```python
from build123d import *
from OCP.BRepFilletAPI import BRepFilletAPI_MakeChamfer

# Parameters (mm, degrees)
SKETCH1_W               = 21
SKETCH1_H               = 36
SKETCH1_R               = 8.9
BOSS_EXTRUDE1_DEPTH     = 24
SKETCH1_2_R             = 8.9
BOSS_EXTRUDE2_DEPTH     = 27
SKETCH2_R               = 2
SKETCH2_R_2             = 1.3
CUT_EXTRUDE1_DEPTH      = 3
CHAMFER1_SIZE           = 4
CHAMFER1_SIZE2          = 2
CHAMFER2_SIZE           = 2
CHAMFER2_SIZE2          = 4
CUT_EXTRUDE2_DEPTH      = 32.784430151
CUT_EXTRUDE2_DEPTH_BACK = 32.784430151
SKETCH4_R               = 2
CUT_EXTRUDE3_DEPTH      = 39.65229618
CUT_EXTRUDE3_DEPTH_BACK = 39.65229618
SKETCH5_W               = 17
SKETCH5_H               = 12.551801511
SKETCH7_W               = 6
SKETCH7_H               = 6
BOSS_EXTRUDE3_DEPTH     = 1.5
BOSS_EXTRUDE4_START     = -21
SKETCH7_2_W             = 6
SKETCH7_2_H             = 6
BOSS_EXTRUDE4_DEPTH     = 1.5
CUT_EXTRUDE6_START      = 1.5
SKETCH6_R               = 2
CUT_EXTRUDE6_DEPTH      = 3
CUT_EXTRUDE7_START      = -19.5
SKETCH6_3_R             = 2
CUT_EXTRUDE7_DEPTH      = 3
SKETCH8_W               = 18
SKETCH8_H               = 10
CUT_EXTRUDE8_DEPTH      = 3
CUT_EXTRUDE9_START      = -21
SKETCH8_2_W             = 18
SKETCH8_2_H             = 10
CUT_EXTRUDE9_DEPTH      = 3


with BuildPart() as part:
    # Sketch1 → Boss-Extrude1 (new body)
    with BuildSketch(Plane.XY):
        Rectangle(SKETCH1_W, SKETCH1_H)
        with Locations((0, 9)):
            Circle(SKETCH1_R, mode=Mode.SUBTRACT)
    extrude(amount=BOSS_EXTRUDE1_DEPTH)

    # Sketch1<2> → Boss-Extrude2 (add)
    with BuildSketch(Plane.XY):
        with Locations((0, 9)):
            Circle(SKETCH1_2_R)
    extrude(amount=BOSS_EXTRUDE2_DEPTH)

    # Sketch2 → Cut-Extrude1 (cut)
    with BuildSketch(Plane.XY.offset(27)):
        with Locations((0, 15)):
            Circle(SKETCH2_R)
        with Locations((6, 9)):
            Circle(SKETCH2_R)
        with Locations((0, 3)):
            Circle(SKETCH2_R)
        with Locations((-6, 9)):
            Circle(SKETCH2_R)
        with Locations((0, 9)):
            Circle(SKETCH2_R_2)
    extrude(amount=-CUT_EXTRUDE1_DEPTH, mode=Mode.SUBTRACT)

    # Chamfer1: one chamfer whose edges measure the first distance from different faces: ONE call of the kernel's chamfer builder (chamfer() names one face for all edges)
    chamfer1_edges_1 = [part.edges().sort_by_distance(p)[0] for p in [
        (-10.5, -18, 12),
    ]]
    chamfer1_side_1 = [part.faces().sort_by_distance(p)[0] for p in [
        (-10.5, 0, 12),
    ]]
    chamfer1_edges_2 = [part.edges().sort_by_distance(p)[0] for p in [
        (10.5, 18, 12),
    ]]
    chamfer1_side_2 = [part.faces().sort_by_distance(p)[0] for p in [
        (10.5, 0, 12),
    ]]
    chamfer1 = BRepFilletAPI_MakeChamfer(part.part.solid().wrapped)
    for e in chamfer1_edges_1:
        chamfer1.Add(CHAMFER1_SIZE, CHAMFER1_SIZE2, e.wrapped, chamfer1_side_1[0].wrapped)  # the first distance lies on this face
    for e in chamfer1_edges_2:
        chamfer1.Add(CHAMFER1_SIZE, CHAMFER1_SIZE2, e.wrapped, chamfer1_side_2[0].wrapped)  # the first distance lies on this face
    add(Compound.cast(chamfer1.Shape()), mode=Mode.REPLACE)

    # Chamfer2: one chamfer whose edges measure the first distance from different faces: ONE call of the kernel's chamfer builder (chamfer() names one face for all edges)
    chamfer2_edges_1 = [part.edges().sort_by_distance(p)[0] for p in [
        (10.5, -18, 12),
    ]]
    chamfer2_side_1 = [part.faces().sort_by_distance(p)[0] for p in [
        (1, -18, 12),
    ]]
    chamfer2_edges_2 = [part.edges().sort_by_distance(p)[0] for p in [
        (-10.5, 18, 12),
    ]]
    chamfer2_side_2 = [part.faces().sort_by_distance(p)[0] for p in [
        (-1, 18, 12),
    ]]
    chamfer2 = BRepFilletAPI_MakeChamfer(part.part.solid().wrapped)
    for e in chamfer2_edges_1:
        chamfer2.Add(CHAMFER2_SIZE, CHAMFER2_SIZE2, e.wrapped, chamfer2_side_1[0].wrapped)  # the first distance lies on this face
    for e in chamfer2_edges_2:
        chamfer2.Add(CHAMFER2_SIZE, CHAMFER2_SIZE2, e.wrapped, chamfer2_side_2[0].wrapped)  # the first distance lies on this face
    add(Compound.cast(chamfer2.Shape()), mode=Mode.REPLACE)

    # Sketch4 → Cut-Extrude2 (cut, two sides: drawn at the far end of the back side and taken through both)
    with BuildSketch(Plane.XY.offset(24).offset(-CUT_EXTRUDE2_DEPTH_BACK)):
        with Locations((0, -15)):
            Circle(SKETCH4_R)
        with Locations((-6, -15)):
            Circle(SKETCH4_R)
        with Locations((6, -15)):
            Circle(SKETCH4_R)
    extrude(amount=CUT_EXTRUDE2_DEPTH + CUT_EXTRUDE2_DEPTH_BACK, mode=Mode.SUBTRACT)

    # Sketch5 → Cut-Extrude3 (cut, two sides: drawn at the far end of the back side and taken through both)
    with BuildSketch(Plane.ZY.offset(10.5).offset(-CUT_EXTRUDE3_DEPTH_BACK)):
        with Locations((12, -19.275900756)):
            Rectangle(SKETCH5_W, SKETCH5_H)
    extrude(amount=CUT_EXTRUDE3_DEPTH + CUT_EXTRUDE3_DEPTH_BACK, mode=Mode.SUBTRACT)

    # Sketch7 → Boss-Extrude3 (add)
    with BuildSketch(Plane(origin=(10.5, 0, 0), x_dir=(0, 0, -1), z_dir=(1, 0, 0))):
        with Locations((-18, 9)):
            Rectangle(SKETCH7_W, SKETCH7_H)
        with Locations((-6, 9)):
            Rectangle(SKETCH7_W, SKETCH7_H)
        with Locations((-6, -9)):
            Rectangle(SKETCH7_W, SKETCH7_H)
        with Locations((-18, -9)):
            Rectangle(SKETCH7_W, SKETCH7_H)
    extrude(amount=BOSS_EXTRUDE3_DEPTH)

    # Sketch7<2> → Boss-Extrude4 (add)
    with BuildSketch(Plane(origin=(10.5, 0, 0), x_dir=(0, 0, -1), z_dir=(1, 0, 0)).offset(BOSS_EXTRUDE4_START)):
        with Locations((-18, 9)):
            Rectangle(SKETCH7_2_W, SKETCH7_2_H)
        with Locations((-6, 9)):
            Rectangle(SKETCH7_2_W, SKETCH7_2_H)
        with Locations((-6, -9)):
            Rectangle(SKETCH7_2_W, SKETCH7_2_H)
        with Locations((-18, -9)):
            Rectangle(SKETCH7_2_W, SKETCH7_2_H)
    extrude(amount=-BOSS_EXTRUDE4_DEPTH)

    # Sketch6 → Cut-Extrude6 (cut)
    with BuildSketch(Plane(origin=(10.5, 0, 0), x_dir=(0, 0, -1), z_dir=(1, 0, 0)).offset(CUT_EXTRUDE6_START)):
        with Locations((-12, 9)):
            Circle(SKETCH6_R)
        with Locations((-6, 9)):
            Circle(SKETCH6_R)
        with Locations((-18, 9)):
            Circle(SKETCH6_R)
        with Locations((-12, -9)):
            Circle(SKETCH6_R)
        with Locations((-6, -9)):
            Circle(SKETCH6_R)
        with Locations((-18, -9)):
            Circle(SKETCH6_R)
    extrude(amount=-CUT_EXTRUDE6_DEPTH, mode=Mode.SUBTRACT)

    # Sketch6<3> → Cut-Extrude7 (cut)
    with BuildSketch(Plane(origin=(10.5, 0, 0), x_dir=(0, 0, -1), z_dir=(1, 0, 0)).offset(CUT_EXTRUDE7_START)):
        with Locations((-12, 9)):
            Circle(SKETCH6_3_R)
        with Locations((-6, 9)):
            Circle(SKETCH6_3_R)
        with Locations((-18, 9)):
            Circle(SKETCH6_3_R)
        with Locations((-12, -9)):
            Circle(SKETCH6_3_R)
        with Locations((-6, -9)):
            Circle(SKETCH6_3_R)
        with Locations((-18, -9)):
            Circle(SKETCH6_3_R)
    extrude(amount=-CUT_EXTRUDE7_DEPTH, mode=Mode.SUBTRACT)

    # Sketch8 → Cut-Extrude8 (cut)
    with BuildSketch(Plane(origin=(10.5, 0, 0), x_dir=(0, 0, -1), z_dir=(1, 0, 0))):
        with Locations((-12, 0)):
            Rectangle(SKETCH8_W, SKETCH8_H)
    extrude(amount=-CUT_EXTRUDE8_DEPTH, mode=Mode.SUBTRACT)

    # Sketch8<2> → Cut-Extrude9 (cut)
    with BuildSketch(Plane(origin=(10.5, 0, 0), x_dir=(0, 0, -1), z_dir=(1, 0, 0)).offset(CUT_EXTRUDE9_START)):
        with Locations((-12, 0)):
            Rectangle(SKETCH8_2_W, SKETCH8_2_H)
    extrude(amount=CUT_EXTRUDE9_DEPTH, mode=Mode.SUBTRACT)


solid = part.part
```
For this review, take the finished solid that the model builds, in its own axes (mm). A direction names the side the tool comes from. Give positions to 0.01 mm unless a question says otherwise; leave off trailing zeros. Order: outer loops, then holes, each group sorted by start corner. A loop starts at its lowest first (then second) coordinate and runs counter-clockwise, first axis right, second up.
1) Take a section at D-D (y = 1.5). Give the boundary of the cut face in (x, z), then the cut area to 3 significant figures.
2) The part is to be moulded in two halves that separate along Y. For faces 6 (the face through (9, 9, 18)), 7 (the face through (-11, 9, 21)), 8 (the face through (0, -18, 2)), say which applies: released by +Y, released by -Y, zero draft, split by the parting line, or undercut.
3) Wall thickness on line 1 (Y direction, x = 0, z = 24.95); line 2 (Y direction, x = 11.25, z = 18); line 3 (Y direction, x = 3, z = 13.75): over which ranges is each line inside the solid? List them lowest first.
4) Take a section at A-A (y = -15). State how many separate pieces and enclosed holes the cut face has, then the cut area to 3 significant figures.
5) For faces 1 (the face through (11, 12, 6)), 2 (the face through (-11, -12, 6)), 3 (the face through (10.521, -7.648, 19.474)), 4 (the face through (-11, -9, 3)), 5 (the face through (11, -9, 15)), list the 3-axis set-ups (+Z, -Z, +X, -X, +Y, -Y) from which the entire face can be reached by the end or side of a thin tool; tool diameter is ignored.
6) Insertion check: pin 1 (1 mm diameter, centred on x = 3.5, y = -10, fed in from +Z); pin 2 (1.5 mm diameter, centred on y = 6.5, z = 22, fed in from +X); pin 3 (1.5 mm diameter, centred on x = -3.5, z = 4.5, fed in from -Y). Each pin has a flat end and moves straight along its axis. Give the tip position at first contact, or say it passes through.
7) Take a section at B-B (x = 6.75). Give the boundary of the cut face in (y, z).
Derived:
1. outline: (-10.5, 0) - (10.5, 0) - (10.5, 3) - (7.5, 3) - (7.5, 21) - (10.5, 21) - (10.5, 24) - (4.79, 24) - (4.79, 27) - (1.32, 27) - (1.32, 24) - (-1.32, 24) - (-1.32, 27) - (-4.79, 27) - (-4.79, 24) - (-10.5, 24) - (-10.5, 21) - (-7.5, 21) - (-7.5, 3) - (-10.5, 3) - close
1. area: 417 mm2
2. face 6: undercut
2. face 7: zero draft
2. face 8: released by -Y
3. line 1: y = 0.1 to 1, 5 to 7.7, 10.3 to 13, 17 to 17.9
3. line 2: y = -12 to -11, -7 to -6, 6 to 7, 11 to 12
3. line 3: y = -13 to 18
4. separate pieces: 8
4. enclosed holes: 0
4. area: 56.0 mm2
5. face 1: +Z, -Z, +X, +Y
5. face 2: +Z, -Z, -X, -Y
5. face 3: +X
5. face 4: -Z, -X, +Y, -Y
5. face 5: +X, +Y, -Y
6. pin 1: stops at z = 24
6. pin 2: stops at x = 10.5
6. pin 3: stops at y = -13
7. outline: (-18, 0) - (-16.85, 0) - (-16.85, 3.5) - (-18, 3.5) - close; (-18, 20.5) - (-16.85, 20.5) - (-16.85, 24) - (-18, 24) - close; (-13.15, 0) - (18, 0) - (18, 24) - (14.8, 24) - (14.8, 27) - (10.85, 27) - (10.85, 24) - (7.15, 24) - (7.15, 27) - (3.2, 27) - (3.2, 24) - (-13.15, 24) - (-13.15, 20.5) - (-13, 20.5) - (-13, 3.5) - (-13.15, 3.5) - close
